Drawing for the job (mm, zero at the part's lowest x, y, z). A direction names the side the tool comes from. Coordinates: 2 decimals unless noted, no trailing zeros. Loops run counter-clockwise (first coordinate to the right, second up) from the corner with the lowest first, then second, coordinate; pieces in that order, holes last. Notation, with made-up numbers: (17.5, 11.5) -> (48.5, 11.5) arc R24 cw to (48.5, 38.5) -> close; hole circle Ø9 at (67.25, -38.75). An arc over 180 degrees is marked (long way). Write item = value, one per line. Start each with the question number.
(1) Tool access for the marked faces 1 and 2: list every direction of +Z, -Z, +X, -X, +Y, -Y with a clear straight run to the whole face (end or side of a thin tool).
(2) Flat gauge pin, fed straight in: P1, Ø8, axis at y = 20.5, z = 15, coming from the +X side. Where does the tip first touch, or does it go through?
(3) Pull direction Z, two halves, no side cores. Call the marked faces 3, 4 and 5: +Z half, -Z half, draft (parallel to the pull), parting line (faces both ways), or undercut.
(4) Drill centre lines: line 1 (Y direction, x = 7, z = 16.5); line 2 (Z direction, x = 16.5, y = 13.75). Where is each one in solid material? Low to high. Write a range as from..to.
(5) Band-saw the part on A-A (z = 7). Write the cut outline in (x, y).
(6) Band-saw the part on C-C (x = 3.75). Write the cut outline in (y, z), and give its area (3 significant figures).
(7) Band-saw the part on B-B (y = 19.5). Write the cut outline in (x, z).
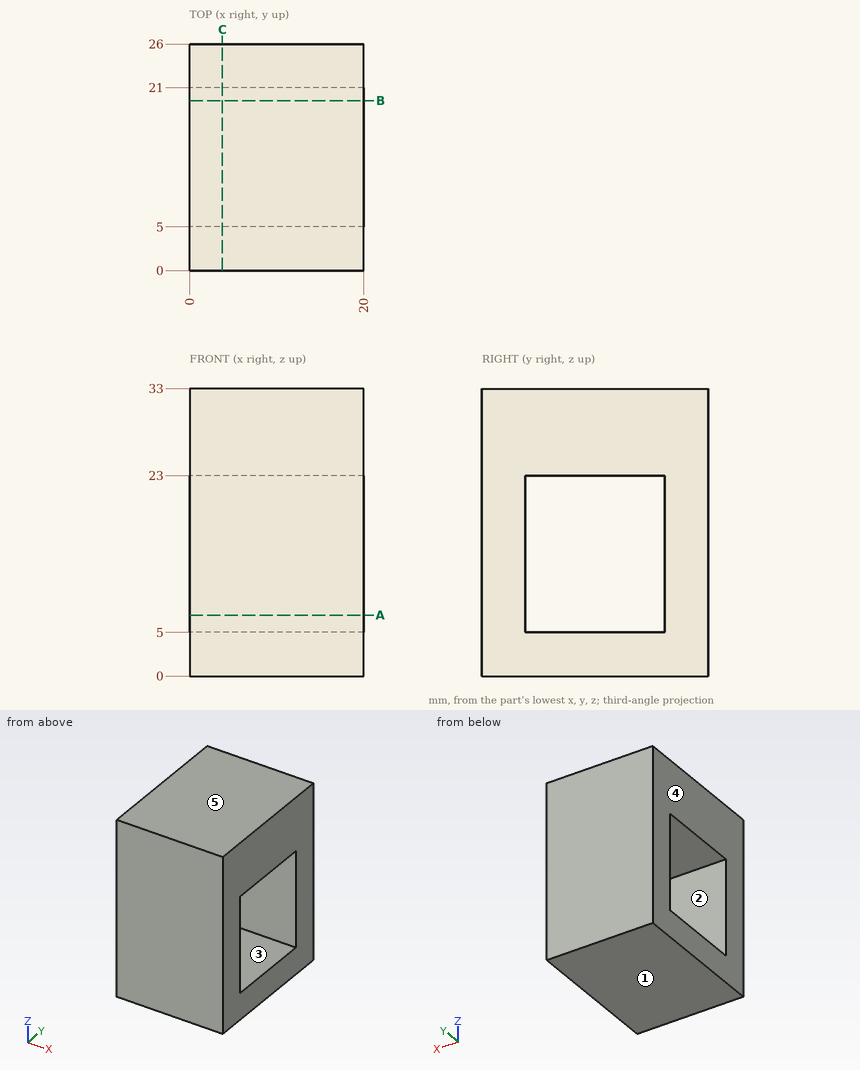
Findings below:
q1.face_1 = -Z, +X, -X, +Y, -Y
q1.face_2 = +X, -X
q2.P1 = 20
q3.face_3 = undercut
q3.face_4 = draft
q3.face_5 = +Z half
q4.line_1 = 0..5, 21..26
q4.line_2 = 0..5, 23..33
q5.outline = (0, 0) -> (20, 0) -> (20, 5) -> (0, 5) -> close; (0, 21) -> (20, 21) -> (20, 26) -> (0, 26) -> close
q6.outline = (0, 0) -> (26, 0) -> (26, 33) -> (0, 33) -> close; hole (5, 5) -> (21, 5) -> (21, 23) -> (5, 23) -> close
q6.area = 570 mm²
q7.outline = (0, 0) -> (20, 0) -> (20, 5) -> (0, 5) -> close; (0, 23) -> (20, 23) -> (20, 33) -> (0, 33) -> close
